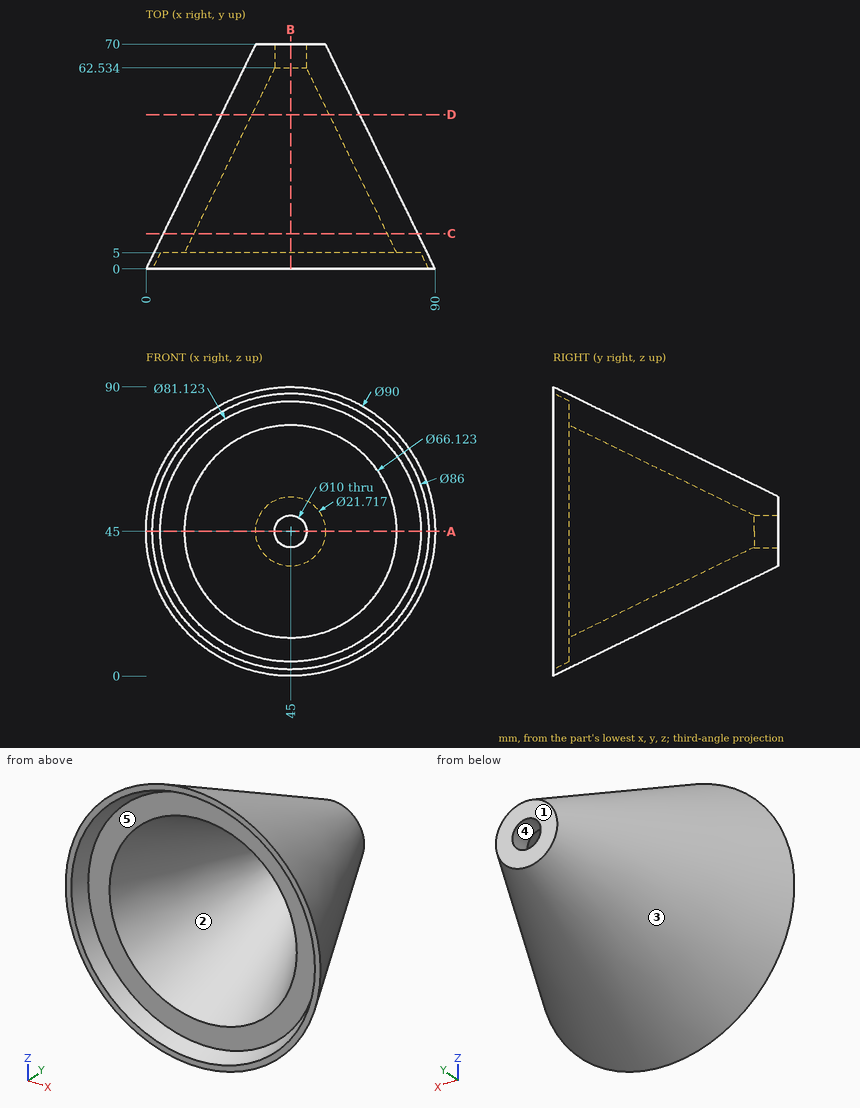
Design review of the part shown in the three views and the two pictorial views. Dimensions are in mm from the part's minimum x, y and z. A direction names the side the tool comes from. Round coordinates to 2 decimals unless told otherwise and drop trailing zeros. Write each loop counter-clockwise with the first axis right and the second up, starting at its lowest first coordinate (ties: lowest second). Pieces come first, ordered by that corner, then holes. Notation, with made-up numbers: (-22, 82) -> (-5, 82) arc R13 ccw to (-5, 104) -> close; hole circle Ø5 at (40.25, 53.25). An arc over 180 degrees is marked (long way). Write item = value, one per line. Start each with the question number.
1) Take a section at D-D, the plane y = 48. State the section outline as (x, z) points, plus the area to 4 significant figures.
2) Mouldability with a two-part tool opening along Z and no side actions: class the marked faces 1, 2 and 3 as +Z half, -Z half, draft (parallel to the pull), parting line (faces both ways), or undercut.
3) Wall thickness on probe 1 along X at (y, z) = (66, 45); probe 2 along X at (y, z) = (17.5, 38) (1 decimal); probe 3 along Z at (x, y) = (47.5, 26): over which ranges is each line inside the solid? List them lowest first. Write a range as from..to.
4) Take a section at C-C, the plane y = 11. State the section outline as (x, z) points (1 decimal), plus the area to 3 significant figures.
5) Take a section at B-B, the plane x = 45. State the section outline as (y, z) points (1 decimal).
6) Tool access review of the marked faces 4 and 5: name each direction out of +Z, -Z, +X, -X, +Y, -Y from which nothing blocks a thin tool from reaching the whole face with its end or side.
7) Take a section at A-A, the plane z = 45. State the section outline as (x, y) points (1 decimal), plus the area to 3 significant figures.
8) Clearance check with flat-ended pins moving along their axes: pin 1 (12 mm diameter, centred on x = 57, y = 59, fed in from -Z) (1 decimal); pin 2 (3 mm diameter, centred on x = 46, z = 21.5, fed in from +Y) (1 decimal); pin 3 (8 mm diameter, centred on x = 54.5, z = 23.5, fed in from +Y) (1 decimal). State where each tip first meets the part, or that it passes through.
Results list:
q1.outline = circle Ø43.18 at (45, 45); hole circle Ø24.18 at (45, 45)
q1.area = 1,005 mm²
q2.face_1 = draft
q2.face_2 = undercut
q2.face_3 = parting line
q3.probe_1 = 32.19..40, 50..57.81
q3.probe_2 = 9.2..19, 71..80.8
q3.probe_3 = 12.78..22.32, 67.68..77.22
q4.outline = circle Ø79.3 at (45, 45); hole circle Ø60.3 at (45, 45)
q4.area = 2,080 mm²
q5.outline = (0, 0) -> (70, 34.1) -> (70, 40) -> (62.5, 40) -> (5, 11.9) -> (5, 4.4) -> (0, 2) -> close; (0, 88) -> (5, 85.6) -> (5, 78.1) -> (62.5, 50) -> (70, 50) -> (70, 55.9) -> (0, 90) -> close
q6.face_4 = +Y, -Y
q6.face_5 = -Y
q7.outline = (0, 0) -> (2, 0) -> (4.4, 5) -> (11.9, 5) -> (40, 62.5) -> (40, 70) -> (34.1, 70) -> close; (50, 62.5) -> (78.1, 5) -> (85.6, 5) -> (88, 0) -> (90, 0) -> (55.9, 70) -> (50, 70) -> close
q7.area = 1,230 mm²
q8.pin_1 = 28.4
q8.pin_2 = 47.1
q8.pin_3 = 52.3
